```python
from build123d import *

# Parameters (mm, degrees)
F0_W     = 62
F0_H     = 25
F1_DEPTH = 25
F2_R     = 3.5
F3_DEPTH = 25
F4_W     = 58
F4_H     = 23
F5_DEPTH = 23
F7_DEPTH = 62.001
F8_R     = 1.5
F9_DEPTH = 2.001


with BuildPart() as f1:
    # F0 (on Top) → F1 (new body)
    with BuildSketch(Plane.XY):
        Rectangle(F0_W, F0_H)
    extrude(amount=F1_DEPTH)

    # F2 (on face) → F3 (cut)
    with BuildSketch(Plane.XZ.offset(12.5)):
        with Locations((0, 12.5)):
            Circle(F2_R)
        with Locations((-15, 12.5)):
            Circle(F2_R)
        with Locations((15, 12.5)):
            Circle(F2_R)
    extrude(amount=-F3_DEPTH, mode=Mode.SUBTRACT)

    # F4 (on face) → F5 (cut)
    with BuildSketch(Plane.XY.offset(25)):
        with Locations((0, 1)):
            Rectangle(F4_W, F4_H)
    extrude(amount=-F5_DEPTH, mode=Mode.SUBTRACT)

    # F6 (on face) → F7 (cut, through all)
    with BuildSketch(Plane.YZ.offset(31)):
        Polygon((12.5, 25), (-10.5, 25), (12.5, 2), align=None)
    extrude(amount=-F7_DEPTH, mode=Mode.SUBTRACT)

    # F8 (on face) → F9 (cut, through all)
    with BuildSketch(Plane.XY.offset(2)):
        with Locations((-25.5, 0)):
            Circle(F8_R)
        with Locations((25.5, 0)):
            Circle(F8_R)
    extrude(amount=-F9_DEPTH, mode=Mode.SUBTRACT)


solid = f1.part
```
Part model, mm, in its own coordinate system. A direction names the side the tool comes from. Round coordinates to 2 decimals unless told otherwise and drop trailing zeros. Write each loop counter-clockwise with the first axis right and the second up, starting at its lowest first coordinate (ties: lowest second). Pieces come first, ordered by that corner, then holes. Notation, with made-up numbers: M -38,-39.75 L 16,-39.75 A34 cw 16,-5.75 Z; hole C 7,13.25 d3. An arc over 180 degrees is marked long. Answer as CSV lines item,"result". Start each with the question number.
1) Band-saw the part on D-D (z = 7.75). List the corners of the cut face in (x, y), then the cut area to 3 significant figures.
2) Drop flat-ended pins along their axis: pin 1 (5 mm diameter, centred on x = 25.5, y = 0, fed in from +Z); pin 2 (9 mm diameter, centred on x = 15, z = 12.5, fed in from +Y). Give the stop position or say it passes through.
3) Band-saw the part on A-A (x = 25.5). List the corners of the cut face in (y, z), then the cut area to 3 significant figures.
4) Which spindle directions (+Z, -Z, +X, -X, +Y, -Y) get a long thin tool onto all of the face, cutting with end or side? Do faces 5 (the face through (0, 0, 0)), 6 (the face through (-0.4, -10.5, 16.2)). Say none if no direction does.
5) Drill centre lines: L1, parallel to X at y = -7, z = 6.5; L2, parallel to Z at x = 15, y = -11; L3, parallel to Y at x = -25.5, z = 0.5. Where is each one in solid material? Low to high.
6) Band-saw the part on B-B (z = 12.5). List the corners of the cut face in (x, y).
7) Band-saw the part on C-C (y = 0). List the corners of the cut face in (x, z).
8) Mould opens along Y. For faces 1 (the face through (24, 0, 1)), 2 (the face through (0, 12.5, 1)), 3 (the face through (0, -12.5, 7)), 4 (the face through (-27, 0, 1)) say: +Y half, -Y half, draft (parallel to the pull), parting line (faces both ways), or undercut.
Worked out:
1,outline,"M -31,-12.5 L 31,-12.5 L 31,6.75 L 29,6.75 L 29,-10.5 L -29,-10.5 L -29,6.75 L -31,6.75 Z"
1,area,"193 mm²"
2,pin 1,"z = 2"
2,pin 2,"y = -10.5"
3,outline,"M -12.5,0 L -1.5,0 L -1.5,2 L -10.5,2 L -10.5,25 L -12.5,25 Z; M 1.5,0 L 12.5,0 L 12.5,2 L 1.5,2 Z"
3,area,"90.0 mm²"
4,face 5,"-Z, +X, -X, +Y, -Y"
4,face 6,"+Z, +Y"
5,L1,"-31 to -29, 29 to 31"
5,L2,"0 to 9, 16 to 25"
5,L3,"-12.5 to -1.5, 1.5 to 12.5"
6,outline,"M -31,-12.5 L -18.5,-12.5 L -18.5,-10.5 L -29,-10.5 L -29,2 L -31,2 Z; M -11.5,-12.5 L -3.5,-12.5 L -3.5,-10.5 L -11.5,-10.5 Z; M 3.5,-12.5 L 11.5,-12.5 L 11.5,-10.5 L 3.5,-10.5 Z; M 18.5,-12.5 L 31,-12.5 L 31,2 L 29,2 L 29,-10.5 L 18.5,-10.5 Z"
7,outline,"M -31,0 L -27,0 L -27,2 L -29,2 L -29,14.5 L -31,14.5 Z; M -24,0 L 24,0 L 24,2 L -24,2 Z; M 27,0 L 31,0 L 31,14.5 L 29,14.5 L 29,2 L 27,2 Z"
8,face 1,"undercut"
8,face 2,"+Y half"
8,face 3,"-Y half"
8,face 4,"undercut"
